Can you work these out from the model? Positions are in its coordinate system, mm. A direction names the side the tool comes from. Round coordinates to 2 decimals unless told otherwise and drop trailing zeros. Loops run counter-clockwise (first coordinate to the right, second up) from the corner with the lowest first, then second, coordinate; pieces in that order, holes last. Notation, with made-up numbers: (78, 75) -> (86, 75) arc R7 ccw to (86, 81) -> close; hole circle Ø1 at (38, -4.75). An arc over 180 degrees is marked (long way). Use a Markdown table: item, result.
from build123d import *

# Parameters (mm, degrees)
BOX022_W          = 47
BOX022_H          = 2
BOX022_DEPTH      = 2
BOX023_W          = 47
BOX023_H          = 2
BOX023_DEPTH      = 2
CYLINDER026_R     = 2
CYLINDER026_DEPTH = 20
CYLINDER025_R     = 2
CYLINDER025_DEPTH = 20
CYLINDER027_R     = 12.5
CYLINDER027_DEPTH = 2.5
CYLINDER023_R     = 4
CYLINDER023_DEPTH = 20
CYLINDER024_R     = 4
CYLINDER024_DEPTH = 20
BOX021_W          = 54
BOX021_H          = 54
BOX021_DEPTH      = 20


with BuildPart() as cube022:
    # Box022 → Box022 (new body)
    with BuildSketch(Plane(origin=(-10, -1, 31), x_dir=(1, 0, 0), z_dir=(0, 0, 1))):
        with Locations((23.5, 1)):
            Rectangle(BOX022_W, BOX022_H)
    extrude(amount=BOX022_DEPTH)


with BuildPart() as cube023:
    # Box023 → Box023 (new body)
    with BuildSketch(Plane(origin=(-10, 25, 31), x_dir=(1, 0, 0), z_dir=(0, 0, 1))):
        with Locations((23.5, 1)):
            Rectangle(BOX023_W, BOX023_H)
    extrude(amount=BOX023_DEPTH)


with BuildPart() as zylinder026:
    # Cylinder026 → Cylinder026 (new body)
    with BuildSketch(Plane(origin=(6, 0, 13), x_dir=(1, 0, 0), z_dir=(0, 0, 1))):
        Circle(CYLINDER026_R)
    extrude(amount=CYLINDER026_DEPTH)


with BuildPart() as fusion013:
    # Cylinder025 → Cylinder025 (new body)
    with BuildSketch(Plane(origin=(-6, 0, 13), x_dir=(1, 0, 0), z_dir=(0, 0, 1))):
        Circle(CYLINDER025_R)
    extrude(amount=CYLINDER025_DEPTH)

    # Fusion013: union Zylinder026
    add(zylinder026.part)


with BuildPart() as zylinder027:
    # Cylinder027 → Cylinder027 (new body)
    with BuildSketch(Plane.XY.offset(13)):
        Circle(CYLINDER027_R)
    extrude(amount=CYLINDER027_DEPTH)


with BuildPart() as zylinder023:
    # Cylinder023 → Cylinder023 (new body)
    with BuildSketch(Plane(origin=(6, 0, 13), x_dir=(1, 0, 0), z_dir=(0, 0, 1))):
        Circle(CYLINDER023_R)
    extrude(amount=CYLINDER023_DEPTH)


with BuildPart() as fusion014:
    # Cylinder024 → Cylinder024 (new body)
    with BuildSketch(Plane(origin=(-6, 0, 13), x_dir=(1, 0, 0), z_dir=(0, 0, 1))):
        Circle(CYLINDER024_R)
    extrude(amount=CYLINDER024_DEPTH)

    # Fusion012: union Zylinder023
    add(zylinder023.part)

    # Fusion014: union Zylinder027
    add(zylinder027.part)


with BuildPart() as cut016:
    # Cut016 base: copy of Fusion014
    add(fusion014.part)

    # Cut016: cut Fusion013
    add(fusion013.part, mode=Mode.SUBTRACT)


with BuildPart() as cut017:
    # Cut017 base: copy of Fusion014
    add(fusion014.part)

    # Cut017: cut Fusion013
    add(fusion013.part, mode=Mode.SUBTRACT)


with BuildPart() as cut017_1:
    # Cut017 placement: moved
    add(cut017.part.moved(Location((26, 0, 0))))


with BuildPart() as cut015:
    # Cut015 base: copy of Fusion014
    add(fusion014.part)

    # Cut015: cut Fusion013
    add(fusion013.part, mode=Mode.SUBTRACT)


with BuildPart() as cut015_1:
    # Cut015 placement: moved
    add(cut015.part.moved(Location((26, 26, 0))))


with BuildPart() as fusion015:
    # Cut014 base: copy of Fusion014
    add(fusion014.part)

    # Cut014: cut Fusion013
    add(fusion013.part, mode=Mode.SUBTRACT)


with BuildPart() as fusion015_1:
    # Cut014 placement: moved
    add(fusion015.part.moved(Location((0, 26, 0))))

    # Fusion015: union Cut016, Cut017, Cut015
    add(cut016.part)
    add(cut017_1.part)
    add(cut015_1.part)


with BuildPart() as obj1:
    # Box021 → Box021 (new body)
    with BuildSketch(Plane(origin=(-14, -14, 13), x_dir=(1, 0, 0), z_dir=(0, 0, 1))):
        with Locations((27, 27)):
            Rectangle(BOX021_W, BOX021_H)
    extrude(amount=BOX021_DEPTH)

    # Cut018: cut Fusion015
    add(fusion015_1.part, mode=Mode.SUBTRACT)

    # Fusion016: union Cube022, Cube023
    add(cube022.part)
    add(cube023.part)


solid = obj1.part
1. I want a section at C-C (x = 6). Please give me the cut outline in (y, z).
Answer sheet:
| item | result |
|---|---|
| outline | (-14, 13) -> (-10.97, 13) -> (-10.97, 15.5) -> (-4, 15.5) -> (-4, 33) -> (-14, 33) -> close; (-2, 13) -> (2, 13) -> (2, 33) -> (-2, 33) -> close; (4, 15.5) -> (10.97, 15.5) -> (10.97, 13) -> (15.03, 13) -> (15.03, 15.5) -> (22, 15.5) -> (22, 33) -> (4, 33) -> close; (24, 13) -> (28, 13) -> (28, 33) -> (24, 33) -> close; (30, 15.5) -> (36.97, 15.5) -> (36.97, 13) -> (40, 13) -> (40, 33) -> (30, 33) -> close |
2. Will these pins go through, and if not, where does the flat tip stop? pin 1 Ø8 at (x, y) = (25, 9) entering from -Z; pin 2 Ø0.6 at (x, y) = (35, 0.5) entering from -Z.
Answer sheet:
| item | result |
|---|---|
| pin 1 | stops at z = 13 |
| pin 2 | stops at z = 31 |
3. Which directions (+Z, -Z, +X, -X, +Y, -Y) give clear straight access to the entire face, cutting with the end or side of a thin tool? Please do faces 1 (the flat face through (-6, 26, 13)), 2 (the flat face through (9, 1, 32)), 3 (the cylindrical face through (18, 26, 23)).
Answer sheet:
| item | result |
|---|---|
| face 1 | -Z, +X, -X, +Y, -Y |
| face 2 | +Z, -Z |
| face 3 | -Z |
4. I need wall thicknesses on line 1 (Y direction, x = 6, z = 22.5); line 2 (Y direction, x = 0, z = 14.6); line 3 (Y direction, x = -3, z = 25.5). Which ranges of each line are inside material? Lowest first, please.
Answer sheet:
| item | result |
|---|---|
| line 1 | y = -14 to -4, -2 to 2, 4 to 22, 24 to 28, 30 to 40 |
| line 2 | y = -14 to -12.5, 12.5 to 13.5, 38.5 to 40 |
| line 3 | y = -14 to -2.65, 2.65 to 23.35, 28.65 to 40 |
5. I want a section at D-D (y = 31.5). Please give me the cut outline in (x, z).
Answer sheet:
| item | result |
|---|---|
| outline | (-14, 13) -> (-11.22, 13) -> (-11.22, 15.5) -> (11.22, 15.5) -> (11.22, 13) -> (14.78, 13) -> (14.78, 15.5) -> (37.22, 15.5) -> (37.22, 13) -> (40, 13) -> (40, 33) -> (-14, 33) -> close |
6. If we mould it in two halves opening along Y, with no side actions, what happens to faces 4 (the cylindrical face through (9.815, 27.201, 24.127)), 5 (the flat face through (6, 0, 13))? For each: +Y half, -Y half, draft (parallel to the pull), parting line (faces both ways), or undercut.
Answer sheet:
| item | result |
|---|---|
| face 4 | undercut |
| face 5 | draft |
7. I want a section at B-B (x = 26). Please give me the cut outline in (y, z), plus the area to 3 significant figures.
Answer sheet:
| item | result |
|---|---|
| outline | (-14, 13) -> (-12.5, 13) -> (-12.5, 15.5) -> (12.5, 15.5) -> (12.5, 13) -> (13.5, 13) -> (13.5, 15.5) -> (38.5, 15.5) -> (38.5, 13) -> (40, 13) -> (40, 33) -> (-14, 33) -> close |
| area | 955 mm² |
8. I want a section at A-A (z = 29). State how many separate pieces and enclosed holes the cut face has, plus the area to 3 significant figures.
Answer sheet:
| item | result |
|---|---|
| separate pieces | 9 |
| enclosed holes | 8 |
| area | 2,610 mm² |
